Could you check a few things on this drawing? It's one solid part, dimensions in mm from its lowest x, y, z. Give positions to 0.01 mm unless a question says otherwise; leave off trailing zeros. Loops run counter-clockwise (first coordinate to the right, second up) from the corner with the lowest first, then second, coordinate; pieces in that order, holes last. Notation, with made-up numbers: M 63.5,62 L 67.5,62 A6 ccw 67.5,72 Z; hole C 36.5,-5 d9. An arc over 180 degrees is marked long. Answer as CSV lines item,"result". Start each with the question number.
Item 1: I want a section at A-A on x = 41.5. List the corners of the cut face in (y, z) for me (1 decimal).
Item 2: If I drill on line 1 along Y through (x, z) = (24.5, 6) (1 decimal); line 2 along X through (y, z) = (63, 8), over which ranges is the centre line in solid material (lowest first)? Write a range as from..to.
Item 3: Will this pin go through, and if not, where does the flat tip stop? P1, Ø4, axis at x = 42.5, y = 62, coming from the +Z side.
Item 4: I want a section at B-B on z = 6.25. List the corners of the cut face in (x, y) for me (1 decimal).
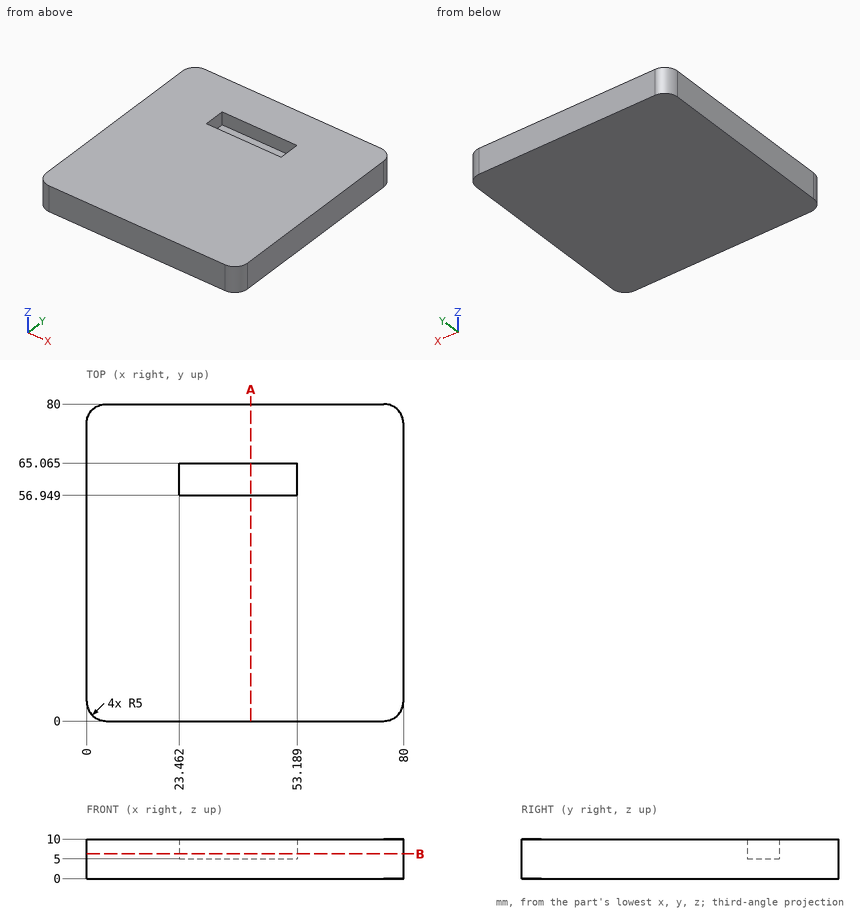
Result:
1,outline,"M 0,0 L 80,0 L 80,10 L 65.1,10 L 65.1,5 L 56.9,5 L 56.9,10 L 0,10 Z"
2,line 1,"0..56.9, 65.1..80"
2,line 2,"0..23.46, 53.19..80"
3,P1,"z = 5"
4,outline,"M 0,5 A5 ccw 5,0 L 75,0 A5 ccw 80,5 L 80,75 A5 ccw 75,80 L 5,80 A5 ccw 0,75 Z; hole M 23.5,56.9 L 53.2,56.9 L 53.2,65.1 L 23.5,65.1 Z"
